Read the model definition and answer for the solid it produces. Units are mm, in the model's axes. A direction names the side the tool comes from. Give positions to 0.01 mm unless a question says otherwise; leave off trailing zeros. Write each loop counter-clockwise with the first axis right and the second up, starting at its lowest first coordinate (ties: lowest second). Pieces come first, ordered by that corner, then holes. Notation, with made-up numbers: M 84,17.5 L 120,17.5 A15 ccw 120,21.5 Z; hole C 63,-1 d6. An arc over 180 degrees is marked long. Use a Markdown table: item, result. Add a question column.
Item 1: The mould has two halves that part along X. Classify faces 1 (the flat face through (30, 2, 141)), 2 (the flat face through (111, 2, 134)), 3 (the flat face through (80, 2, 141)), 4 (the flat face through (10, 2, 141)): pulls with the +X half, pulls with the -X half, needs draft (parallel to the pull), parting line crosses it, or undercut.
Item 2: Given P1, Ø1.5, axis at y = 2, z = 139.5, coming from the +X side; P2, Ø1, axis at y = 3.5, z = 72.5, coming from the -X side; P3, Ø0.9, axis at y = 3, z = 140, coming from the -X side, each flat-ended and moving along its own axis, determine where each tip first touches the part or whether it passes through.
Item 3: For faces 5 (the flat face through (44, 2, 0)), 6 (the flat face through (74, 3, -6)), 7 (the flat face through (90, 2, 141)), 8 (the flat face through (-3, 2, 134)), 9 (the flat face through (114, 3, 127)), determine the directions among +Z, -Z, +X, -X, +Y, -Y from which every point of the face is accessible in a straight line to the end or side of a thin tool.
Item 4: A cutting plane is placed at B-B on x = 63. Determine the outline of the cut face in (y, z), then the cut area to 3 significant figures.
Item 5: Consider probe 1 along X at (y, z) = (2.4, 116); probe 2 along Z at (x, y) = (8, 3.7); probe 3 along Z at (x, y) = (-1, 2.6). Determine where each line is inside the solid, lowest interval first. Write a range as [from, to].
Item 6: A cutting plane is placed at A-A on z = 22. Determine the outline of the cut face in (x, y), then the cut area to 3 significant figures.
from build123d import *

# Parameters (mm, degrees)
SKETCH_1_W          = 108
SKETCH_1_H          = 138
EXTRUDE_1_DEPTH     = 4
SKETCH_3_W          = 108
SKETCH_3_H          = 138
CUT_EXTRUDE_2_DEPTH = 1
SKETCH_4_W          = 10
SKETCH_4_H          = 3
EXTRUDE_2_DEPTH     = 6
SKETCH_5_W          = 10
SKETCH_5_H          = 3
SKETCH_5_W_2        = 15
EXTRUDE_3_DEPTH     = 6
SKETCH_6_W          = 15
SKETCH_6_H          = 3
SKETCH_6_W_2        = 10
EXTRUDE_4_DEPTH     = 6
SKETCH_7_W          = 10
SKETCH_7_H          = 3
EXTRUDE_5_DEPTH     = 6


with BuildPart() as part:
    # Эскиз1 → Бобышка-Вытянуть1 (new body)
    with BuildSketch(Plane(origin=(0, 0, 0), x_dir=(1, 0, 0), z_dir=(0, 1, 0))):
        with Locations((54, -69)):
            Rectangle(SKETCH_1_W, SKETCH_1_H)
    extrude(amount=EXTRUDE_1_DEPTH)

    # Эскиз3 → Вырез-Вытянуть2 (cut)
    with BuildSketch(Plane.XZ):
        with Locations((54, 69)):
            Rectangle(SKETCH_3_W, SKETCH_3_H)
    extrude(amount=-CUT_EXTRUDE_2_DEPTH, mode=Mode.SUBTRACT)

    # Эскиз4 → Бобышка-Вытянуть2 (add)
    with BuildSketch(Plane.XY.offset(138)):
        with Locations((15, 2.5)):
            Rectangle(SKETCH_4_W, SKETCH_4_H)
        with Locations((35, 2.5)):
            Rectangle(SKETCH_4_W, SKETCH_4_H)
        with Locations((55, 2.5)):
            Rectangle(SKETCH_4_W, SKETCH_4_H)
        with Locations((75, 2.5)):
            Rectangle(SKETCH_4_W, SKETCH_4_H)
        with Locations((95, 2.5)):
            Rectangle(SKETCH_4_W, SKETCH_4_H)
    extrude(amount=EXTRUDE_2_DEPTH)

    # Эскиз5 → Бобышка-Вытянуть3 (add)
    with BuildSketch(Plane.ZY):
        with Locations((14, 2.5)):
            Rectangle(SKETCH_5_W, SKETCH_5_H)
        with Locations((126.5, 2.5)):
            Rectangle(SKETCH_5_W_2, SKETCH_5_H)
    extrude(amount=EXTRUDE_3_DEPTH)

    # Эскиз6 → Бобышка-Вытянуть4 (add)
    with BuildSketch(Plane(origin=(108, 0, 0), x_dir=(0, 0, -1), z_dir=(1, 0, 0))):
        with Locations((-126.5, 2.5)):
            Rectangle(SKETCH_6_W, SKETCH_6_H)
        with Locations((-14, 2.5)):
            Rectangle(SKETCH_6_W_2, SKETCH_6_H)
    extrude(amount=EXTRUDE_4_DEPTH)

    # Эскиз7 → Бобышка-Вытянуть5 (add)
    with BuildSketch(Plane(origin=(0, 0, 0), x_dir=(-1, 0, 0), z_dir=(0, 0, -1))):
        with Locations((-94, 2.5)):
            Rectangle(SKETCH_7_W, SKETCH_7_H)
        with Locations((-74, 2.5)):
            Rectangle(SKETCH_7_W, SKETCH_7_H)
        with Locations((-54, 2.5)):
            Rectangle(SKETCH_7_W, SKETCH_7_H)
        with Locations((-34, 2.5)):
            Rectangle(SKETCH_7_W, SKETCH_7_H)
        with Locations((-14, 2.5)):
            Rectangle(SKETCH_7_W, SKETCH_7_H)
    extrude(amount=EXTRUDE_5_DEPTH)


solid = part.part
Filled in:
| question | item | result |
|---|---|---|
| 1 | face 1 | undercut |
| 1 | face 2 | needs draft |
| 1 | face 3 | undercut |
| 1 | face 4 | pulls with the -X half |
| 2 | P1 | x = 100 |
| 2 | P2 | x = 0 |
| 2 | P3 | x = 10 |
| 3 | face 5 | -Z, +Y, -Y |
| 3 | face 6 | -Z, +X, -X, +Y, -Y |
| 3 | face 7 | +Z, +Y, -Y |
| 3 | face 8 | +Z, -X, +Y, -Y |
| 3 | face 9 | +Z, -Z, +X, +Y, -Y |
| 4 | outline | M 1,0 L 4,0 L 4,138 L 1,138 Z |
| 4 | area | 414 mm² |
| 5 | probe 1 | [0, 108] |
| 5 | probe 2 | [0, 138] |
| 5 | probe 3 | [9, 19], [119, 134] |
| 6 | outline | M 0,1 L 108,1 L 108,4 L 0,4 Z |
| 6 | area | 324 mm² |
